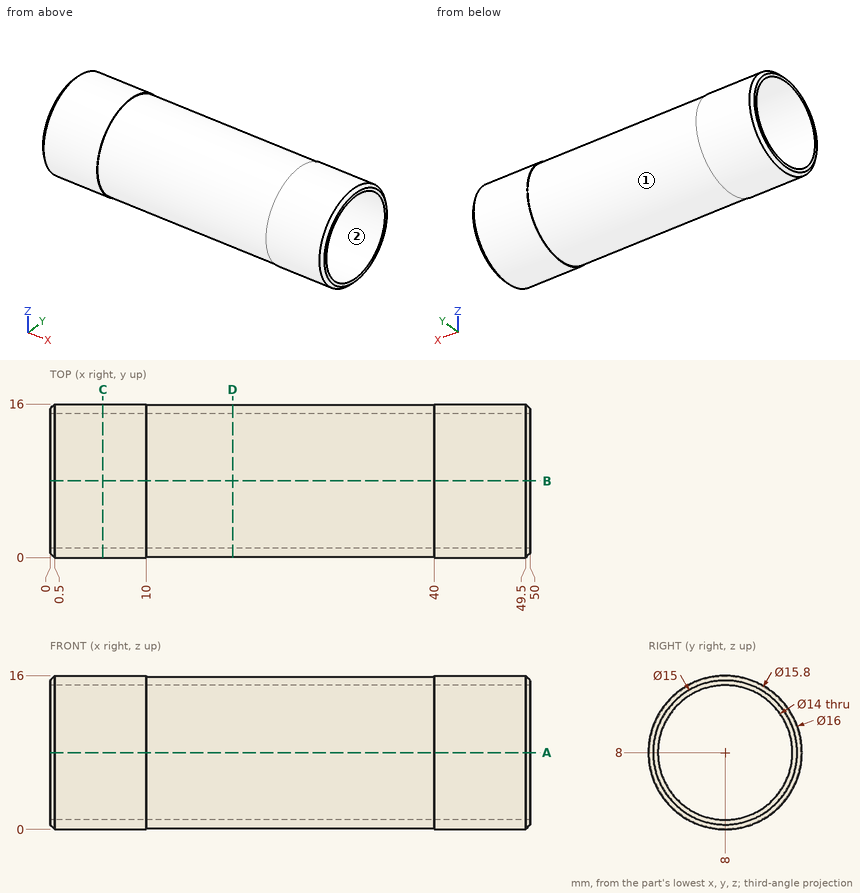
Drawing for the job (mm, zero at the part's lowest x, y, z). Round coordinates to 2 decimals unless told otherwise and drop trailing zeros. Order: outer loops, then holes, each group sorted by start corner. A loop starts at its lowest first (then second) coordinate and runs counter-clockwise, first axis right, second up.
Item 1: Mould opens along Y. For the marked faces 1 and 2 say: pulls with the +Y half, pulls with the -Y half, needs draft (parallel to the pull), parting line crosses it, or undercut.
Item 2: Saw through at D-D on x = 19. Write the cut outline in (y, z), then the cut area to 3 significant figures.
Item 3: Pin check, flat tips, straight feed: pin 1 (5 mm diameter, centred on x = 42.5, y = 3, fed in from +Z); pin 2 (5 mm diameter, centred on x = 38.5, z = 13, fed in from +Y); pin 3 (3 mm diameter, centred on x = 6.5, z = 5, fed in from -Y); pin 4 (8.5 mm diameter, centred on y = 8, z = 8, fed in from -X). Stop position of each tip, or through.
Item 4: Saw through at A-A on z = 8. Write the cut outline in (x, y), then the cut area to 3 significant figures.
Item 5: Saw through at C-C on x = 5.5. Write the cut outline in (y, z), then the cut area to 3 significant figures.
Item 6: Probe line 1 along Z through (x, y) = (29, 8); line 2 along Y through (x, z) = (42, 7.75). List the from-to ranges inside material, lowest first.
Reported:
1. face 1: parting line crosses it
1. face 2: undercut
2. outline: circle Ø15.8 at (8, 8); hole circle Ø14 at (8, 8)
2. area: 42.1 mm2
3. pin 1: stops at z = 15.6
3. pin 2: stops at y = 15.49
3. pin 3: stops at y = 0.14
3. pin 4: passes through
4. outline: (0, 0.5) - (0.5, 0) - (10, 0) - (10, 0.1) - (40, 0.1) - (40, 0) - (49.5, 0) - (50, 0.5) - (50, 1) - (0, 1) - close; (0, 15) - (50, 15) - (50, 15.5) - (49.5, 16) - (40, 16) - (40, 15.9) - (10, 15.9) - (10, 16) - (0.5, 16) - (0, 15.5) - close
4. area: 93.5 mm2
5. outline: circle Ø16 at (8, 8); hole circle Ø14 at (8, 8)
5. area: 47.1 mm2
6. line 1: z = 0.1 to 1, 15 to 15.9
6. line 2: y = 0 to 1, 15 to 16
